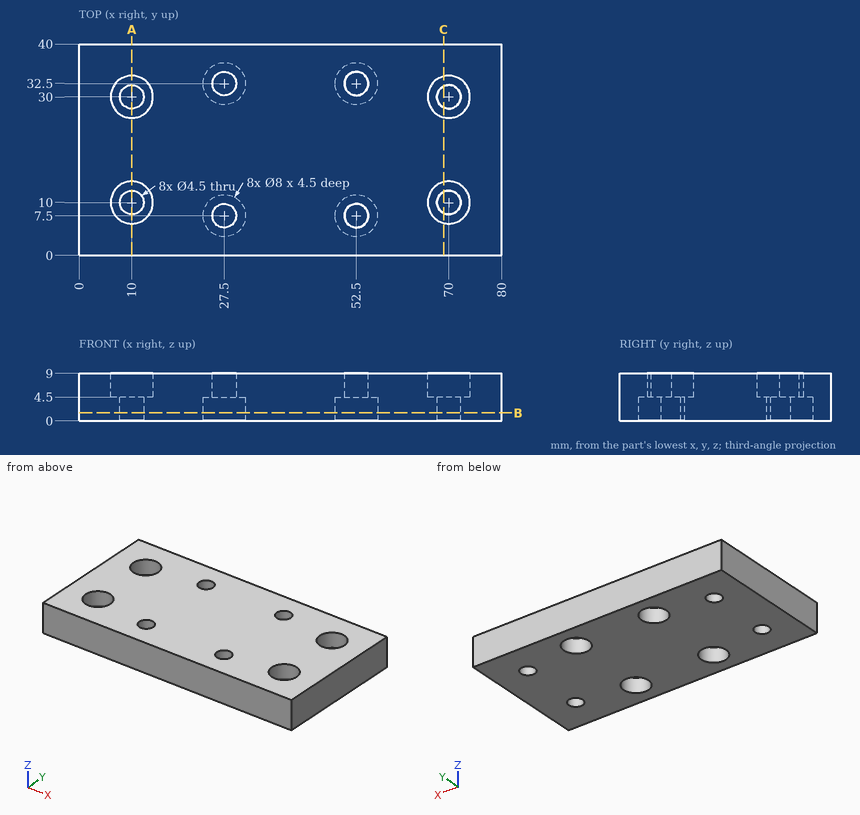
The drawing under review shows one solid part. Ordinate dimensions are in mm from its lowest x, y, z. Round coordinates to 2 decimals unless told otherwise and drop trailing zeros. Write each loop counter-clockwise with the first axis right and the second up, starting at its lowest first coordinate (ties: lowest second). Pieces come first, ordered by that corner, then holes. Notation, with made-up numbers: (52.25, 14) - (70.25, 14) arc R37 cw to (70.25, 52) - close; hole circle Ø6 at (-32.5, 73). An arc over 180 degrees is marked (long way). Use one line per item in the form item = value.
Q1. For line 1 (Y direction, x = 52.5, z = 5.8); line 2 (Y direction, x = 70, z = 5); line 3 (X direction, y = 29.5, z = 4), list the stretches that pass through material, from the lowest coordinate up. Write a range as [from, to].
Answer key:
line_1 = [0, 5.25], [9.75, 30.25], [34.75, 40]
line_2 = [0, 6], [14, 26], [34, 40]
line_3 = [0, 7.81], [12.19, 24.85], [30.15, 49.85], [55.15, 67.81], [72.19, 80]
Q2. Insertion check: pin 1 Ø10.5 at (x, y) = (10, 10) entering from -Z; pin 2 Ø2.5 at (x, y) = (71.5, 9.5) entering from +Z; pin 3 Ø7 at (x, y) = (52.5, 32.5) entering from -Z. Each pin has a flat end and moves straight along its axis. Give the tip position at first contact, or say it passes through.
Answer key:
pin_1 = 0
pin_2 = 4.5
pin_3 = 4.5
Q3. Consider section B-B (z = 1.5). State how many separate pieces and enclosed holes the cut face has, and give its area (3 significant figures).
Answer key:
separate_pieces = 1
enclosed_holes = 8
area = 2,940 mm2
Q4. Consider section A-A (x = 10). State the section outline as (y, z) points.
Answer key:
outline = (0, 0) - (7.75, 0) - (7.75, 4.5) - (6, 4.5) - (6, 9) - (0, 9) - close; (12.25, 0) - (27.75, 0) - (27.75, 4.5) - (26, 4.5) - (26, 9) - (14, 9) - (14, 4.5) - (12.25, 4.5) - close; (32.25, 0) - (40, 0) - (40, 9) - (34, 9) - (34, 4.5) - (32.25, 4.5) - close
Q5. Consider section C-C (x = 69). State the section outline as (y, z) points.
Answer key:
outline = (0, 0) - (7.98, 0) - (7.98, 4.5) - (6.13, 4.5) - (6.13, 9) - (0, 9) - close; (12.02, 0) - (27.98, 0) - (27.98, 4.5) - (26.13, 4.5) - (26.13, 9) - (13.87, 9) - (13.87, 4.5) - (12.02, 4.5) - close; (32.02, 0) - (40, 0) - (40, 9) - (33.87, 9) - (33.87, 4.5) - (32.02, 4.5) - close
